```python
from build123d import *

# Parameters (mm, degrees)
F0_W     = 30
F0_H     = 30
F1_DEPTH = 25
F2_T     = -2
F3_R     = 0.25
F4_R     = 2.2673190991
F5_DEPTH = 25.001


with BuildPart() as f1:
    # F0 (on Top) → F1 (new body)
    with BuildSketch(Plane.XY):
        Rectangle(F0_W, F0_H)
    extrude(amount=F1_DEPTH)

    # F2
    f2_openings = [f1.faces().sort_by_distance(p)[0] for p in [
        (0, 0, 25),
    ]]
    offset(amount=F2_T, openings=f2_openings)

    # F3
    f3_edges = [f1.edges().sort_by_distance(p)[0] for p in [
        (0, 13, 25),
        (-13, 13, 13.5),
        (0, 13, 2),
        (13, 13, 13.5),
        (-13, 0, 25),
        (-13, -13, 13.5),
        (-13, 0, 2),
        (0, -13, 25),
        (13, -13, 13.5),
        (0, -13, 2),
        (13, 0, 25),
        (13, 0, 2),
        (0, -15, 0),
        (15, 0, 0),
        (0, 15, 0),
        (-15, 0, 0),
        (-15, -15, 12.5),
        (15, -15, 12.5),
        (0, -15, 25),
        (15, 15, 12.5),
        (-15, 15, 12.5),
        (0, 15, 25),
        (-15, 0, 25),
        (15, 0, 25),
    ]]
    fillet(f3_edges, radius=F3_R)

    # F4 (on face) → F5 (cut, through all)
    with BuildSketch(Plane(origin=(0, 0, 0), x_dir=(1, 0, 0), z_dir=(0, 0, -1))):
        Circle(F4_R)
    extrude(amount=-F5_DEPTH, mode=Mode.SUBTRACT)


solid = f1.part
```
Geometry check sheet. Reference: the model listing, model coordinates, mm. A direction names the side the tool comes from. Coordinates: 2 decimals unless noted, no trailing zeros. Order: outer loops, then holes, each group sorted by start corner. A loop starts at its lowest first (then second) coordinate and runs counter-clockwise, first axis right, second up. Notation, with made-up numbers: (-21, 52) - (10, 52) arc R21 ccw to (10, 63) - close; hole circle Ø5 at (19.5, 66). An arc over 180 degrees is marked (long way). Answer as a JSON object with one key per item and string values. Group by question number.
Item 1: Depth check by flat-ended pin: pin 1 Ø13 at (x, y) = (2.5, -3.5) entering from +Z; pin 2 Ø6 at (x, y) = (0, 0) entering from -Z. Enter the tip coordinate at first touch or a pass-through.
Item 2: Tool access check on faces 1 (the face through (-13, 0, 13)), 2 (the face through (15, 0, 12)). Record the directions out of +Z, -Z, +X, -X, +Y, -Y that give a thin tool (end or side, any length) a straight path to the whole face; none if there is none.
Item 3: Scan lines: probe 1 along X at (y, z) = (0, 0.6); probe 2 along Y at (x, z) = (-3, 13.5). Record each from-to range of solid material in increasing order.
Item 4: Sectioned sample at C-C, the plane z = 14.5. Record the cut outline in (x, y), and give its area (3 significant figures).
Item 5: Sectioned sample at A-A, the plane x = 0. Record the cut outline in (y, z), and give its area (3 significant figures).
Item 6: Draft check along X on faces 3 (the face through (3, 0, 2)), 4 (the face through (-14, 0, 25)), 5 (the face through (-15, 0, 12)). Enter one of: +X half, -X half, draft (parallel to the pull), parting line (faces both ways), or undercut.
Item 7: Sectioned sample at D-D, the plane y = 10.75. Record the cut outline in (x, z), and give its area (3 significant figures).
Resolved:
{
 "1": {"pin 1": "z = 2", "pin 2": "z = 0"},
 "2": {"face 1": "+Z", "face 2": "+Z, -Z, +X, +Y, -Y"},
 "3": {"probe 1": "-15 to -2.27, 2.27 to 15", "probe 2": "-15 to -13, 13 to 15"},
 "4": {"outline": "(-15, -14.75) arc R0.25 ccw to (-14.75, -15) - (14.75, -15) arc R0.25 ccw to (15, -14.75) - (15, 14.75) arc R0.25 ccw to (14.75, 15) - (-14.75, 15) arc R0.25 ccw to (-15, 14.75) - close; hole (-13, -12.75) arc R0.25 ccw to (-12.75, -13) - (12.75, -13) arc R0.25 ccw to (13, -12.75) - (13, 12.75) arc R0.25 ccw to (12.75, 13) - (-12.75, 13) arc R0.25 ccw to (-13, 12.75) - close", "area": "224 mm^2"},
 "5": {"outline": "(-15, 0.25) arc R0.25 ccw to (-14.75, 0) - (-2.27, 0) - (-2.27, 2) - (-12.75, 2) arc R0.25 cw to (-13, 2.25) - (-13, 24.75) arc R0.25 ccw to (-13.25, 25) - (-14.75, 25) arc R0.25 ccw to (-15, 24.75) - close; (2.27, 0) - (14.75, 0) arc R0.25 ccw to (15, 0.25) - (15, 24.75) arc R0.25 ccw to (14.75, 25) - (13.25, 25) arc R0.25 ccw to (13, 24.75) - (13, 2.25) arc R0.25 cw to (12.75, 2) - (2.27, 2) - close", "area": "143 mm^2"},
 "6": {"face 3": "undercut", "face 4": "draft", "face 5": "-X half"},
 "7": {"outline": "(-15, 0.25) arc R0.25 ccw to (-14.75, 0) - (14.75, 0) arc R0.25 ccw to (15, 0.25) - (15, 24.75) arc R0.25 ccw to (14.75, 25) - (13.25, 25) arc R0.25 ccw to (13, 24.75) - (13, 2.25) arc R0.25 cw to (12.75, 2) - (-12.75, 2) arc R0.25 cw to (-13, 2.25) - (-13, 24.75) arc R0.25 ccw to (-13.25, 25) - (-14.75, 25) arc R0.25 ccw to (-15, 24.75) - close", "area": "152 mm^2"}
}
